Check sheet for the drawn part. Datum: minimum x, y, z corner. Units: mm. A direction names the side the tool comes from. Round coordinates to 2 decimals unless told otherwise and drop trailing zeros. Write each loop counter-clockwise with the first axis right and the second up, starting at its lowest first coordinate (ties: lowest second). Pieces come first, ordered by that corner, then holes. Notation, with made-up numbers: (-11.75, 17.5) - (40.25, 17.5) arc R33 cw to (40.25, 45.5) - close; hole circle Ø8 at (62, -6). An arc over 180 degrees is marked (long way). Answer as a JSON object with one key per item and string values.
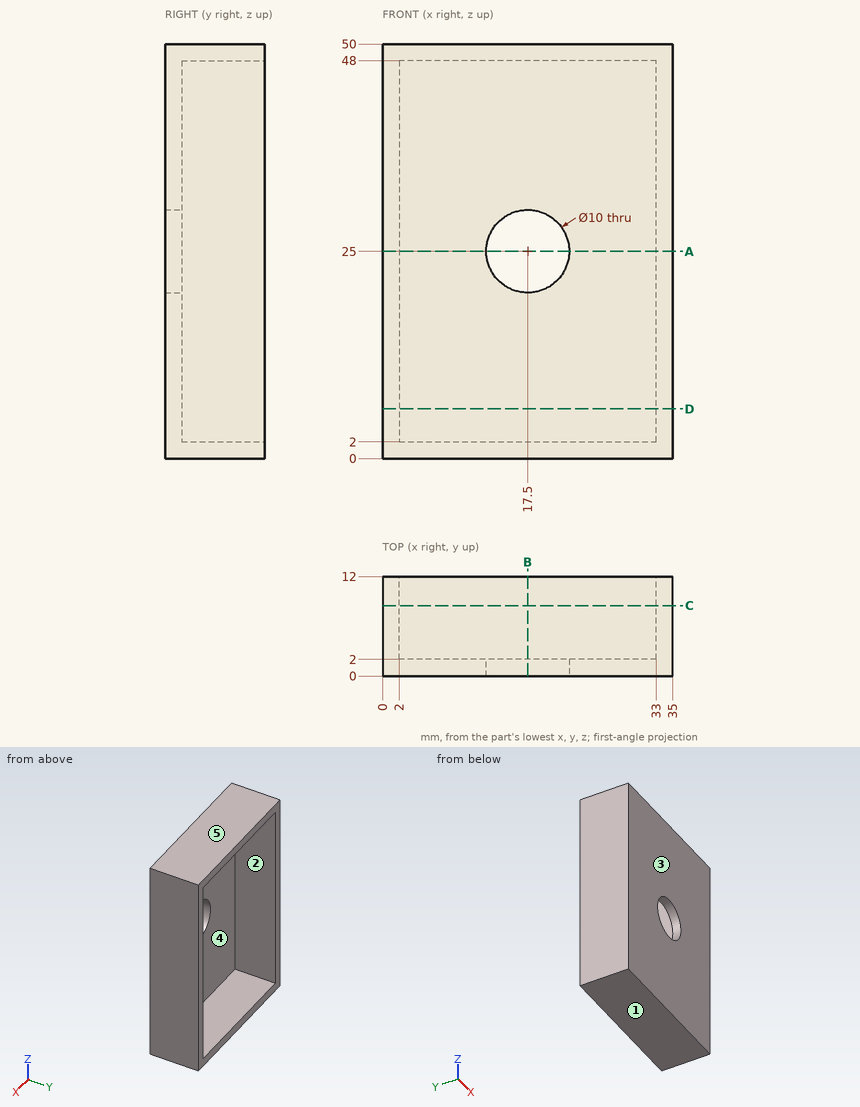
1. Cross-section at B-B (x = 17.5). Record the boundary of the cut face in (y, z), plus the area to 3 significant figures.
Completed:
{"outline": "(0, 0) - (12, 0) - (12, 2) - (2, 2) - (2, 20) - (0, 20) - close; (0, 30) - (2, 30) - (2, 48) - (12, 48) - (12, 50) - (0, 50) - close", "area": "120 mm^2"}
2. Access from +Z, -Z, +X, -X, +Y, -Y to the whole of each face (thin tool, end or side, straight path). Record for the marked faces 1 and 2.
Completed:
{"face 1": "-Z, +X, -X, +Y, -Y", "face 2": "+Y"}
3. Go/stop test with a flat-tipped pin: pin 1 (10 mm diameter, centred on x = 25.5, z = 31, fed in from +Y). Record where the tip stops, or that it passes through.
Completed:
{"pin 1": "stops at y = 2"}
4. Cross-section at C-C (y = 8.5). Record the boundary of the cut face in (x, z), plus the area to 3 significant figures.
Completed:
{"outline": "(0, 0) - (35, 0) - (35, 50) - (0, 50) - close; hole (2, 2) - (33, 2) - (33, 48) - (2, 48) - close", "area": "324 mm^2"}
5. Mould release check, pull along Z, two halves, no side actions. Record for the marked faces 3, 4 and 5: released by +Z, released by -Z, zero draft, split by the parting line, or undercut.
Completed:
{"face 3": "zero draft", "face 4": "undercut", "face 5": "released by +Z"}
6. Cross-section at D-D (z = 6). Record the boundary of the cut face in (x, y), plus the area to 3 significant figures.
Completed:
{"outline": "(0, 0) - (35, 0) - (35, 12) - (33, 12) - (33, 2) - (2, 2) - (2, 12) - (0, 12) - close", "area": "110 mm^2"}
7. Cross-section at A-A (z = 25). Record the boundary of the cut face in (x, y), plus the area to 3 significant figures.
Completed:
{"outline": "(0, 0) - (12.5, 0) - (12.5, 2) - (2, 2) - (2, 12) - (0, 12) - close; (22.5, 0) - (35, 0) - (35, 12) - (33, 12) - (33, 2) - (22.5, 2) - close", "area": "90.0 mm^2"}
8. Material ranges on probe 1 along Z at (x, y) = (19, 9.5); probe 2 along X at (y, z) = (11, 46.5); probe 3 along Z at (x, y) = (17.5, 0.95), recorded low to high. Write a range as from..to.
Completed:
{"probe 1": "z = 0..2, 48..50", "probe 2": "x = 0..2, 33..35", "probe 3": "z = 0..20, 30..50"}
